Could you check a few things on this model? Use its own coordinates, in mm. A direction names the side the tool comes from. Give positions to 0.01 mm unless a question says otherwise; leave off trailing zeros. Loops run counter-clockwise (first coordinate to the right, second up) from the corner with the lowest first, then second, coordinate; pieces in that order, holes last.
1. I need wall thicknesses on line 1 along Z through (x, y) = (1.5, 5); line 2 along Y through (x, z) = (1.25, 1.85); line 3 along Y through (x, z) = (-3, 1.85). Which ranges of each line are inside material? Lowest first, please.
2. Imagine slicing it at A-A (z = 2.3). Count the separate pieces of the cut face and the enclosed holes in it, plus the area to 3 significant figures.
3. Imagine slicing it at B-B (z = 1.2). List the corners of the cut face in (x, y) for me.
4. For P1, Ø1.8, axis at x = 1.5, y = 6.5, coming from the +Z side; P2, Ø1.5, axis at x = 4, z = 1.5, coming from the +Y side; P3, Ø0.7, axis at y = -8.5, z = 2.5, coming from the -X side, each with a flat end and sliding along its axis, tell me the tip position at first contact or that it passes through.
5. For faces 5 (the flat face through (6.76, 4.15, 2.19)), 6 (the flat face through (-5, 0, 2.6)), 7 (the flat face through (-7.004, -0.385, 2.194)), 8 (the flat face through (-3, -3.3, 2.2)), which set-ups out of +Z, -Z, +X, -X, +Y, -Y let a thin tool reach every point of the face, with its end or its side?
6. Thinking about a two-plate mould opening in Y: for faces 1 (the flat face through (-6.911, -5.655, 2.194)), 2 (the flat face through (-6.46, 4.42, 2.19)), 3 (the flat face through (3.144, 1.176, 2.194)), 4 (the flat face through (1, 0, 2.6)), which applies, +Y half, -Y half, draft (parallel to the pull), parting line (faces both ways), or undercut?
```python
from build123d import *

# Parameters (mm, degrees)
F3_DEPTH = 0.8


with BuildPart() as f1:
    # F0 (on Front) → F1 (revolve)
    with BuildSketch(Plane.XZ):
        Polygon((0, 1.8), (-10.7, 1.8), (-10.7, 0.4530665231), (-9.0727129846, 0), (0, 0), align=None)
    revolve(axis=Axis((0, 0, 1.1966938619), (0, 0, -1)))

    # F2 (on face) → F3 (join)
    with BuildSketch(Plane.XY.offset(1.8)):
        with BuildLine():
            add(Edge.make_bspline(
                [(-1.6867941013, 8.8509330526), (0.8566841716, 8.8753895834), (2.649315499, 9.0611870259), (4.7208145261, 7.7993022278), (5.050977692, 6.6498457454)],
                knots=[0, 0, 0, 0, 0.5589307471, 1, 1, 1, 1], degree=3))
            Line((-1.6867941013, 8.8509330526), (-1.6867941013, 8.5329981521))
            add(Edge.make_bspline(
                [(-1.6867941013, 8.5329981521), (-1.3774677293, 8.5470557254), (-0.6938875858, 8.5771007031), (-0.6173685214, 7.6472761807), (-0.6112642586, 7.1267476305)],
                knots=[0, 0, 0, 0, 0.441787592, 1, 1, 1, 1], degree=3))
            Line((-0.6112642586, 7.1267476305), (-0.6112642586, 0.3177910403))
            Line((-0.6112642586, 0.3177910403), (-4.9199624918, 3.8612245116))
            add(Edge.make_bspline(
                [(-4.9199624918, 3.8612245116), (-5.1154879855, 4.0527227146), (-5.5120993261, 4.4411649455), (-5.1191776451, 4.8610289061), (-4.9199624918, 5.0739040598)],
                knots=[0, 0, 0, 0, 0.4929901738, 1, 1, 1, 1], degree=3))
            Line((-4.9199624918, 5.0739040598), (-5.3968969733, 5.457715597))
            Line((-5.3968969733, 5.457715597), (-7.5489841402, 3.3604586497))
            Line((-7.5489841402, 3.3604586497), (-7.0966347121, 3.000701312))
            add(Edge.make_bspline(
                [(-7.0966347121, 3.000701312), (-6.8613198471, 3.1750743352), (-6.4010215426, 3.5161645889), (-5.9145178984, 3.2846312905), (-5.6767258793, 3.1714630313)],
                knots=[0, 0, 0, 0, 0.5112225325, 1, 1, 1, 1], degree=3))
            Line((-5.6767258793, 3.1714630313), (-0.6559019093, -0.6086938665))
            Line((-0.6559019093, -0.6086938665), (-5.8705802076, -4.3306946754))
            add(Edge.make_bspline(
                [(-5.8705802076, -4.3306946754), (-6.1822484494, -4.5196679636), (-6.7864429099, -4.8860081888), (-7.308925656, -4.5013103723), (-7.5618904084, -4.3150554411)],
                knots=[0, 0, 0, 0, 0.5158409455, 1, 1, 1, 1], degree=3))
            Line((-7.5618904084, -4.3150554411), (-7.9826125875, -4.6550915577))
            Line((-7.9826125875, -4.6550915577), (-5.8098412119, -6.6837798804))
            Line((-5.8098412119, -6.6837798804), (-5.3775920533, -6.3379807398))
            add(Edge.make_bspline(
                [(-5.4053300992, -5.1254965365), (-5.5515290524, -5.3446676224), (-5.8379925252, -5.7741133125), (-5.5289246402, -6.1526388002), (-5.3775920533, -6.3379807398)],
                knots=[0, 0, 0, 0, 0.5103580985, 1, 1, 1, 1], degree=3))
            Line((-5.4053300992, -5.1254965365), (-0.6126278895, -1.4923192712))
            Line((-0.6126278895, -1.4923192712), (-0.6126278895, -7.048912812))
            add(Edge.make_bspline(
                [(-0.6126278895, -7.048912812), (-0.6389726569, -7.377813444), (-0.6916788554, -8.0358227462), (-1.3219282839, -8.234017122), (-1.637152629, -8.3331456408)],
                knots=[0, 0, 0, 0, 0.4998419184, 1, 1, 1, 1], degree=3))
            Line((-1.637152629, -8.3331456408), (-1.637152629, -8.9842546731))
            Line((-1.637152629, -8.9842546731), (1.6732236836, -8.9842546731))
            Line((1.6732236836, -8.9842546731), (1.6732236836, -8.2714613527))
            add(Edge.make_bspline(
                [(0.4535702465, -7.048912812), (0.4870410433, -7.3872676951), (0.5558033707, -8.0823831835), (1.2942327078, -8.2073324667), (1.6732236836, -8.2714613527)],
                knots=[0, 0, 0, 0, 0.4867606733, 1, 1, 1, 1], degree=3))
            Line((0.4535702465, -7.048912812), (0.4535702465, -1.4659117442))
            Line((0.4535702465, -1.4659117442), (4.8928316683, -5.2557615563))
            add(Edge.make_bspline(
                [(4.8928316683, -5.2557615563), (5.103411153, -5.4165492766), (5.3978362889, -6.0029897915), (5.1020476496, -6.4001318691), (4.9510909234, -6.6109133504)],
                knots=[0, 0, 0, 0, 0.5154207237, 1, 1, 1, 1], degree=3))
            Line((4.9510909234, -6.6109133504), (5.3739010935, -7.0078365295))
            Line((5.3739010935, -7.0078365295), (7.4263224378, -4.8215580173))
            Line((7.4263224378, -4.8215580173), (7.0269443095, -4.4466322288))
            add(Edge.make_bspline(
                [(5.4299915209, -4.4800881296), (5.7073067114, -4.6913712485), (6.2579025081, -5.1108635847), (6.7718523941, -4.6669584172), (7.0269443095, -4.4466322288)],
                knots=[0, 0, 0, 0, 0.5036638351, 1, 1, 1, 1], degree=3))
            Line((5.4299915209, -4.4800881296), (0.4608821182, -0.5992884981))
            Line((0.4608821182, -0.5992884981), (5.9025837108, 3.000701312))
            add(Edge.make_bspline(
                [(5.9025837108, 3.000701312), (6.1652393352, 3.1131659914), (6.6968427958, 3.3407895685), (7.1827875665, 2.993159634), (7.4286358431, 2.8172873426)],
                knots=[0, 0, 0, 0, 0.4940818558, 1, 1, 1, 1], degree=3))
            Line((7.4286358431, 2.8172873426), (7.8171929345, 3.1411375385))
            Line((7.8171929345, 3.1411375385), (5.6788134389, 5.183564499))
            Line((5.6788134389, 5.183564499), (5.1636509597, 4.7825793736))
            add(Edge.make_bspline(
                [(5.1636509597, 4.7825793736), (5.3563745653, 4.5959784132), (5.7323232052, 4.2319733033), (5.3994815796, 3.8708627719), (5.23726549, 3.6948693451)],
                knots=[0, 0, 0, 0, 0.5126328046, 1, 1, 1, 1], degree=3))
            Line((5.23726549, 3.6948693451), (0.4013032594, 0.3040304291))
            Line((0.4013032594, 0.3040304291), (0.4013032594, 3.9351717569))
            add(Edge.make_bspline(
                [(5.050977692, 6.6498457454), (5.2227766775, 5.7417653934), (3.8530424976, 4.1063453678), (1.8400062355, 3.7766705272), (0.4013032594, 3.9351717569)],
                knots=[0, 0, 0, 0, 0.4558296962, 1, 1, 1, 1], degree=3))
        make_face()
        with BuildLine():
            Line((0.3797819663, 4.424153241), (0.3797819663, 8.4475489607))
            add(Edge.make_bspline(
                [(0.3797819663, 8.4475489607), (2.7214622988, 8.8398724894), (5.0507446574, 6.4596899692), (2.9288335052, 3.8387254341), (0.3797819663, 4.424153241)],
                knots=[0, 0, 0, 0, 0.5012880833, 1, 1, 1, 1], degree=3))
        make_face(mode=Mode.SUBTRACT)
        Polygon((-6.2060756609, 1.6079591587), (-7.8247580677, -2.4339009542), (-6.9814925082, -2.4339009542), (-6.5453206189, -1.1932341149), (-6.0219140723, -2.0558852702), (-5.2755754441, -1.1932341149), (-4.9654087052, -2.5017498992), (-3.7344344892, -2.5017498992), (-5.2755754441, 1.6079591587), align=None)
        Polygon((-6.3382112782, -0.5918067245), (-5.9152944013, 0.4642193671), (-5.4694297723, -0.6213641609), (-5.9734508395, -1.2998539023), align=None, mode=Mode.SUBTRACT)
        with BuildLine():
            Line((4.3641445227, -2.3708629888), (5.8277440257, -2.3417847697))
            add(Edge.make_bspline(
                [(5.8277440257, -2.3417847697), (5.1487722105, -0.2610644891), (4.6605925288, 0.2992301122), (5.9169845073, 0.9749441024), (7.2274061463, 0.3335519894), (6.3030754531, -1.3617813756), (5.9440564364, -2.3223995231)],
                knots=[0, 0, 0, 0, 0.3215656024, 0.5011300693, 0.686712218, 1, 1, 1, 1], degree=3))
            Line((5.9440564364, -2.3223995231), (7.3494995013, -2.3999412078))
            Line((7.3494995013, -2.3999412078), (7.7662859112, -1.5372899361))
            Line((7.7662859112, -1.5372899361), (6.8939416669, -1.7020660453))
            add(Edge.make_bspline(
                [(4.8681655899, -1.6923733056), (3.9570508525, -0.8103366708), (3.8497648676, 1.987677069), (7.9298202319, 1.7446883295), (7.8729055822, -0.6455606199), (6.8939416669, -1.7020660453)],
                knots=[0, 0, 0, 0, 0.3420298118, 0.6610694697, 1, 1, 1, 1], degree=3))
            Line((4.8681655899, -1.6923733056), (4.0636705235, -1.5857535182))
            Line((4.0636705235, -1.5857535182), (4.3641445227, -2.3708629888))
        make_face()
    extrude(amount=F3_DEPTH)


solid = f1.part
```
Derived:
1. line 1: z = 0 to 1.8
1. line 2: y = -8.98 to -8.19, -2.15 to -1.22, -0.08 to 0.9, 3.88 to 4.29, 8.52 to 8.88
1. line 3: y = -3.3 to -2.28, 1.16 to 2.28
2. separate pieces: 3
2. enclosed holes: 2
2. area: 77.0 mm2
3. outline: circle Ø21.4 at (0, 0)
4. P1: stops at z = 1.8
4. P2: stops at y = 10.19
4. P3: stops at x = -1.64
5. face 5: +Z, +X, +Y
5. face 6: +Z, +X, -X, +Y, -Y
5. face 7: +Z, -X
5. face 8: +Z
6. face 1: -Y half
6. face 2: +Y half
6. face 3: undercut
6. face 4: draft
